from build123d import *

# Parameters (mm, degrees)
SKETCH2_R           = 1.75
SKETCH2_W           = 13.5
SKETCH2_H           = 3.5
BOSS_EXTRUDE2_DEPTH = 12
BOSS_EXTRUDE3_START = 7
SKETCH2_4_R         = 1.75
SKETCH2_4_W         = 13.5
SKETCH2_4_H         = 6.5
SKETCH2_4_H_2       = 3.5
BOSS_EXTRUDE3_DEPTH = 5
CUT_EXTRUDE1_START  = 12
SKETCH2_6_W         = 13.5
SKETCH2_6_H         = 1.5
CUT_EXTRUDE1_DEPTH  = 5.5
FILLET1_R           = 4.5
CUT_EXTRUDE4_DEPTH  = 5
BOSS_EXTRUDE4_DEPTH = 5
FILLET2_R           = 1


with BuildPart() as part:
    # Sketch2 → Boss-Extrude2 (new body)
    with BuildSketch(Plane(origin=(0, 0, 0), x_dir=(1, 0, 0), z_dir=(0, 1, 0))):
        with BuildLine():
            Line((-20, 12.5), (-20, -12.5))
            Line((-20, -12.5), (-7.5, -12.5))
            ThreePointArc((-7.5, -12.5), (-5.732233047, -13.232233047), (-5, -15))
            Line((-5, -15), (-5, -15.5))
            ThreePointArc((-5, -15.5), (0, -20.5), (5, -15.5))
            Line((5, -15.5), (5, -15))
            ThreePointArc((5, -15), (5.732233047, -13.232233047), (7.5, -12.5))
            Line((7.5, -12.5), (20, -12.5))
            Line((20, -12.5), (20, -5))
            Line((20, -5), (26, -5))
            Line((26, -5), (26, 5))
            Line((26, 5), (20, 5))
            Line((20, 5), (20, 12.5))
            Line((20, 12.5), (7.5, 12.5))
            ThreePointArc((7.5, 12.5), (5.732233047, 13.232233047), (5, 15))
            Line((5, 15), (5, 15.5))
            ThreePointArc((5, 15.5), (0, 20.5), (-5, 15.5))
            Line((-5, 15.5), (-5, 15))
            ThreePointArc((-5, 15), (-5.732233047, 13.232233047), (-7.5, 12.5))
            Line((-7.5, 12.5), (-20, 12.5))
        make_face()
        with Locations(Location((0, -15.5, 0), (0, 0, 270))):
            Circle(SKETCH2_R, mode=Mode.SUBTRACT)
        with Locations(Location((0, 15.5, 0), (0, 0, 270))):
            Circle(SKETCH2_R, mode=Mode.SUBTRACT)
        with Locations((8.75, 0)):
            Rectangle(SKETCH2_W, SKETCH2_H, mode=Mode.SUBTRACT)
    extrude(amount=BOSS_EXTRUDE2_DEPTH)

    # Sketch2<4> → Boss-Extrude3 (add)
    with BuildSketch(Plane(origin=(0, 0, 0), x_dir=(1, 0, 0), z_dir=(0, 1, 0)).offset(BOSS_EXTRUDE3_START)):
        with BuildLine():
            Line((-20, -12.5), (-7.5, -12.5))
            ThreePointArc((-7.5, -12.5), (-5.732233047, -13.232233047), (-5, -15))
            Line((-5, -15), (-5, -15.5))
            ThreePointArc((-5, -15.5), (0, -20.5), (5, -15.5))
            Line((5, -15.5), (5, -15))
            ThreePointArc((5, -15), (5.732233047, -13.232233047), (7.5, -12.5))
            Line((7.5, -12.5), (20, -12.5))
            Line((20, -12.5), (20, -5))
            Line((20, -5), (26, -5))
            Line((26, -5), (26, 5))
            Line((26, 5), (20, 5))
            Line((20, 5), (20, 12.5))
            Line((20, 12.5), (7.5, 12.5))
            ThreePointArc((7.5, 12.5), (5.732233047, 13.232233047), (5, 15))
            Line((5, 15), (5, 15.5))
            ThreePointArc((5, 15.5), (0, 20.5), (-5, 15.5))
            Line((-5, 15.5), (-5, 15))
            ThreePointArc((-5, 15), (-5.732233047, 13.232233047), (-7.5, 12.5))
            Line((-7.5, 12.5), (-20, 12.5))
            Line((-20, 12.5), (-20, -12.5))
        make_face()
        with Locations(Location((0, -15.5, 0), (0, 0, 270))):
            Circle(SKETCH2_4_R, mode=Mode.SUBTRACT)
        with Locations(Location((0, 15.5, 0), (0, 0, 270))):
            Circle(SKETCH2_4_R, mode=Mode.SUBTRACT)
        with Locations((8.75, 0)):
            Rectangle(SKETCH2_4_W, SKETCH2_4_H, mode=Mode.SUBTRACT)
        with Locations((8.75, 0)):
            Rectangle(SKETCH2_4_W, SKETCH2_4_H_2, mode=Mode.SUBTRACT)
    extrude(amount=BOSS_EXTRUDE3_DEPTH)

    # Sketch2<6> → Cut-Extrude1 (cut)
    with BuildSketch(Plane(origin=(0, 0, 0), x_dir=(1, 0, 0), z_dir=(0, 1, 0)).offset(CUT_EXTRUDE1_START)):
        with Locations((8.75, -2.5)):
            Rectangle(SKETCH2_6_W, SKETCH2_6_H)
        with Locations((8.75, 2.5)):
            Rectangle(SKETCH2_6_W, SKETCH2_6_H)
    extrude(amount=-CUT_EXTRUDE1_DEPTH, mode=Mode.SUBTRACT)

    # Fillet1
    fillet1_edges = [part.edges().sort_by_distance(p)[0] for p in [
        (20, 6, -5),
        (20, 6, 5),
    ]]
    fillet(fillet1_edges, radius=FILLET1_R)

    # Sketch3 → Cut-Extrude4 (cut)
    with BuildSketch(Plane.XZ):
        Polygon((7.930232558, 10.25), (2, 1.75), (15.5, 1.75), (15.5, 12.5), (9.5, 12.5), align=None)
        Polygon((2, 10.25), (2, 1.75), (7.930232558, 10.25), align=None)
    extrude(amount=-CUT_EXTRUDE4_DEPTH, mode=Mode.SUBTRACT)

    # Sketch4 → Boss-Extrude4 (add)
    with BuildSketch(Plane(origin=(0, 12, 0), x_dir=(1, 0, 0), z_dir=(0, 1, 0))):
        with BuildLine():
            Line((-5, 11.375), (5, 11.375))
            ThreePointArc((5, 11.375), (7.5, 8.875), (5, 6.375))
            Line((5, 6.375), (-5, 6.375))
            ThreePointArc((-5, 6.375), (-7.5, 8.875), (-5, 11.375))
        make_face()
        with BuildLine():
            Line((-5, -11.375), (5, -11.375))
            ThreePointArc((5, -11.375), (7.5, -8.875), (5, -6.375))
            Line((5, -6.375), (-5, -6.375))
            ThreePointArc((-5, -6.375), (-7.5, -8.875), (-5, -11.375))
        make_face()
    extrude(amount=BOSS_EXTRUDE4_DEPTH)

    # Fillet2
    fillet2_edges = [part.edges().sort_by_distance(p)[0] for p in [
        (-7.5, 17, -8.875),
        (0, 17, -6.375),
        (7.5, 17, -8.875),
        (0, 17, -11.375),
        (-7.5, 17, 8.875),
        (0, 17, 11.375),
        (7.5, 17, 8.875),
        (0, 17, 6.375),
    ]]
    fillet(fillet2_edges, radius=FILLET2_R)


solid = part.part
Work out the finished part from the listing and answer in its coordinate system (mm). A direction names the side the tool comes from. Coordinates: 2 decimals unless noted, no trailing zeros. Write each loop counter-clockwise with the first axis right and the second up, starting at its lowest first coordinate (ties: lowest second). Pieces come first, ordered by that corner, then holes. Notation, with made-up numbers: (-39, -36) - (2, -36) arc R24 cw to (2, -11) - close; hole circle Ø5 at (48.25, -21.75). An arc over 180 degrees is marked (long way). One line per question, with ' | ' between items.
1) Find section C-C, the plane y = 11. Determine the outline of the cut face in (x, z), and give its area (3 significant figures).
Checks:
outline: (-20, -12.5) - (-7.5, -12.5) arc R2.5 cw to (-5, -15) - (-5, -15.5) arc R5 ccw to (5, -15.5) - (5, -15) arc R2.5 cw to (7.5, -12.5) - (20, -12.5) - (20, -9.5) arc R4.5 cw to (24.5, -5) - (26, -5) - (26, 5) - (24.5, 5) arc R4.5 cw to (20, 9.5) - (20, 12.5) - (7.5, 12.5) arc R2.5 cw to (5, 15) - (5, 15.5) arc R5 ccw to (-5, 15.5) - (-5, 15) arc R2.5 cw to (-7.5, 12.5) - (-20, 12.5) - close; hole circle Ø3.5 at (0, -15.5); hole circle Ø3.5 at (0, 15.5); hole (2, -3.25) - (15.5, -3.25) - (15.5, 3.25) - (2, 3.25) - close | area: 1,110 mm2
2) For faces 5 (the face through (-14, 6, -12.5)), 6 (the face through (9, 6.5, -3)), 7 (the face through (-0.07, 16.7, -6.66)), 8 (the face through (25, 6, -5)), determine the directions among +Z, -Z, +X, -X, +Y, -Y from which every point of the face is accessible in a straight line to the end or side of a thin tool.
Checks:
face 5: -Z, -X, +Y, -Y | face 6: +Y | face 7: +X, -X, +Y | face 8: -Z, +X, +Y, -Y
3) Find section A-A, the plane y = 3. Give the number of separate pieces and of enclosed holes in the cut face, and give its area (3 significant figures).
Checks:
separate pieces: 1 | enclosed holes: 2 | area: 1,020 mm2
4) Flat-ended cylindrical pins translate along their axes: P1, Ø8, axis at x = 12.5, z = -9, coming from the +Y side; P2, Ø0.8, axis at x = 25.5, y = 8, coming from the -Z side; P3, Ø8, axis at x = 6, y = 4, coming from the -Z side. Find the tip coordinate at first contact, or state that the pin passes through.
Checks:
P1: y = 12 | P2: z = -5 | P3: z = -20.08
5) Find section B-B, the plane x = 0. Determine the outline of the cut face in (y, z) (3 decimals), and give its area (3 significant figures).
Checks:
outline: (0, -20.5) - (12, -20.5) - (12, -17.25) - (0, -17.25) - close; (0, -13.75) - (12, -13.75) - (12, -11.375) - (16, -11.375) arc R1 ccw to (17, -10.375) - (17, -7.375) arc R1 ccw to (16, -6.375) - (12, -6.375) - (12, 6.375) - (16, 6.375) arc R1 ccw to (17, 7.375) - (17, 10.375) arc R1 ccw to (16, 11.375) - (12, 11.375) - (12, 13.75) - (0, 13.75) - close; (0, 17.25) - (12, 17.25) - (12, 20.5) - (0, 20.5) - close | area: 457 mm2
6) Find section D-D, the plane x = -10.5. Determine the outline of the cut face in (y, z), and give its area (3 significant figures).
Checks:
outline: (0, -12.5) - (12, -12.5) - (12, 12.5) - (0, 12.5) - close | area: 300 mm2
7) The mould has two halves that part along X. Classify faces 1 (the face through (20, 6, 11)), 2 (the face through (0.526, 5.916, -13.831)), 3 (the face through (-14, 6, 12.5)), 4 (the face through (-7.5, 14, 8.8)): +X half, -X half, draft (parallel to the pull), parting line (faces both ways), or undercut.
Checks:
face 1: +X half | face 2: undercut | face 3: draft | face 4: -X half
8) Consider probe 1 along X at (y, z) = (8, 15.5); probe 2 along X at (y, z) = (8.75, -2); probe 3 along Z at (x, y) = (-1, 6.5). Determine where each line is inside the solid, lowest interval first. Write a range as [from, to].
Checks:
probe 1: [-5, -1.75], [1.75, 5] | probe 2: [-20, 2], [15.5, 26] | probe 3: [-20.4, -16.94], [-14.06, 14.06], [16.94, 20.4]
